Geometry: final body of the model. Coordinates: model frame, mm. Round coordinates to 2 decimals unless told otherwise and drop trailing zeros. Loops run counter-clockwise (first coordinate to the right, second up) from the corner with the lowest first, then second, coordinate; pieces in that order, holes last. Notation, with made-up numbers: (53.25, 58) -> (112.25, 58) arc R25 cw to (112.25, 96) -> close; hole circle Ø7 at (41, 3). An arc over 180 degrees is marked (long way). Answer in a Markdown table with one row per item.
```python
from build123d import *

# Parameters (mm, degrees)
F1_DEPTH = 60
F3_DEPTH = 30
F5_D     = 12
F7_DEPTH = 10
F9_D     = 10


with BuildPart() as f1:
    # F0 (on Right) → F1 (new body)
    with BuildSketch(Plane.YZ):
        Polygon((-296.18248, 422.540385), (-346.18248, 422.540385), (-346.18248, -227.459615), (-296.18248, -227.459615), (-296.18248, -175.331955), (353.81752, -175.331955), (353.81752, -125.331955), (-296.18248, -125.331955), align=None)
    extrude(amount=F1_DEPTH)

    # F2 (on face) → F3 (cut)
    with BuildSketch(Plane(origin=(0, 0, 0), x_dir=(0, -1, 0), z_dir=(-1, 0, 0))):
        Polygon((346.18248, -125.331955), (-353.81752, -125.331955), (-353.81752, -165.331955), (-323.81752, -165.331955), (-323.81752, -145.331955), (306.18248, -145.331955), (306.18248, -165.331955), (346.18248, -165.331955), align=None)
    extrude(amount=-F3_DEPTH, mode=Mode.SUBTRACT)

    # F5 (through all)
    with Locations(Plane(origin=(30, 0, 0), x_dir=(0, -1, 0), z_dir=(-1, 0, 0))):
        with Locations((-338.81752, -145.331955), (326.18248, -145.331955)):
            Hole(F5_D / 2)

    # F6 (on face) → F7 (cut)
    with BuildSketch(Plane(origin=(0, -296.18248, 0), x_dir=(-1, 0, 0), z_dir=(0, 1, 0))):
        Polygon((-30, 364.668045), (-30, -125.331955), (-20, -125.331955), (-20, 364.668045), (0, 364.668045), (0, 374.668045), (0, 422.540385), (-40, 422.540385), (-40, 364.668045), align=None)
    extrude(amount=-F7_DEPTH, mode=Mode.SUBTRACT)

    # F9 (through all)
    with Locations(Plane(origin=(0, -306.18248, 0), x_dir=(-1, 0, 0), z_dir=(0, 1, 0))):
        with Locations((-25, 407.540385)):
            Hole(F9_D / 2)


solid = f1.part
```
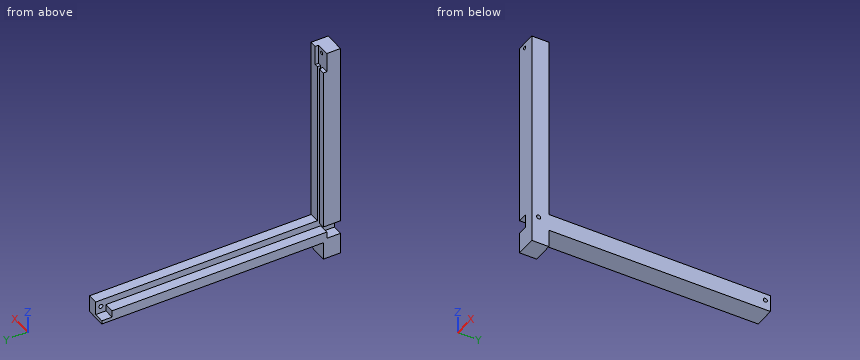
Item 1: Cut plane C-C (y = -72.5). Output: boundary loops of the cut face in (x, z).
Answer:
| item | result |
|---|---|
| outline | (0, -175.33) -> (60, -175.33) -> (60, -125.33) -> (30, -125.33) -> (30, -145.33) -> (0, -145.33) -> close |
Item 2: Line query: probe 1 along Z at (x, y) = (25, -320); probe 2 along Y at (x, z) = (37.5, 163.5); probe 3 along Z at (x, y) = (38, 127). Output: solid intervals per line, ascending. Write a range as [from, to].
Answer:
| item | result |
|---|---|
| probe 1 | z = [-227.46, -165.33], [-125.33, 402.54], [412.54, 422.54] |
| probe 2 | y = [-346.18, -296.18] |
| probe 3 | z = [-175.33, -125.33] |
Item 3: Cut plane D-D (z = -41). Output: boundary loops of the cut face in (x, y), then the cut area to 3 significant figures.
Answer:
| item | result |
|---|---|
| outline | (0, -346.18) -> (60, -346.18) -> (60, -296.18) -> (30, -296.18) -> (30, -306.18) -> (20, -306.18) -> (20, -296.18) -> (0, -296.18) -> close |
| area | 2,900 mm² |
Item 4: Cut plane B-B (z = 383). Output: boundary loops of the cut face in (x, y).
Answer:
| item | result |
|---|---|
| outline | (0, -346.18) -> (60, -346.18) -> (60, -296.18) -> (40, -296.18) -> (40, -306.18) -> (0, -306.18) -> close |
Item 5: Pin query (flat end, axial travel): pin 1 Ø3 at (x, y) = (39, 20) entering from +Z; pin 2 Ø19 at (y, z) = (338.82, -145.33) entering from +X; pin 3 Ø5 at (x, y) = (36.5, -301.5) entering from +Z; pin 4 Ø14 at (y, z) = (-326.18, -145.33) entering from -X. Return the tip coordinate at first contact, or that it passes through.
Answer:
| item | result |
|---|---|
| pin 1 | stops at z = -125.33 |
| pin 2 | stops at x = 60 |
| pin 3 | stops at z = 364.67 |
| pin 4 | stops at x = 30 |
Item 6: Cut plane A-A (x = 48). Output: boundary loops of the cut face in (y, z), then the cut area to 3 significant figures.
Answer:
| item | result |
|---|---|
| outline | (-346.18, -227.46) -> (-296.18, -227.46) -> (-296.18, -175.33) -> (353.82, -175.33) -> (353.82, -125.33) -> (-296.18, -125.33) -> (-296.18, 422.54) -> (-346.18, 422.54) -> close; hole circle Ø12 at (-326.18, -145.33); hole circle Ø12 at (338.82, -145.33) |
| area | 64,800 mm² |
